Verification items for the finished model (mm, model axes). Face numbers are marked on the shaded views. A direction names the side the tool comes from. Coordinates: 2 decimals unless noted, no trailing zeros. Order: outer loops, then holes, each group sorted by start corner. A loop starts at its lowest first (then second) coordinate and runs counter-clockwise, first axis right, second up. Notation, with made-up numbers: M -38,20 L 18,20 A6 ccw 18,31 Z; hole C 88.5,45.25 d3. An arc over 180 degrees is marked long. Return JSON: item names as keys, results as strings. Group by question number.
Q1. Section check C-C, the plane z = 15.5. Enter the section's corners in (x, y), then the cut area to 3 significant figures.
Q2. Thickness scan on probe 1 along X at (y, z) = (-7, 20.5); probe 2 along X at (y, z) = (-21.5, 28); probe 3 along Z at (x, y) = (-29, -13). Record the ranges inside material, lowest first.
Q3. Section check B-B, the plane x = -28. Enter the section's corners in (y, z), then the cut area to 3 significant figures.
Q4. Section check D-D, the plane x = -24. Enter the section's corners in (y, z), then the cut area to 3 significant figures.
Q5. Mould release check, pull along X, two halves, no side actions. Record for the marked faces 1, 2 and 3: pulls with the +X half, pulls with the -X half, needs draft (parallel to the pull), parting line crosses it, or undercut.
Q6. Section check A-A, the plane y = -18. Enter the section's corners in (x, z), then the cut area to 3 significant figures.
Q7. Go/stop test with flat-tipped pins: pin 1 Ø4 at (x, z) = (-14, 7.5) entering from +Y; pin 2 Ø19.5 at (y, z) = (-38.5, 24) entering from +X; pin 3 Ø1 at (y, z) = (-32, 13.5) entering from +X; pin 4 Ø2 at (x, z) = (-24.5, 5.5) entering from -Y. Record where each tip stops, or that it passes through.
Q8. Access from +Z, -Z, +X, -X, +Y, -Y to the whole of each face (thin tool, end or side, straight path). Record for the marked faces 4, 5 and 6.
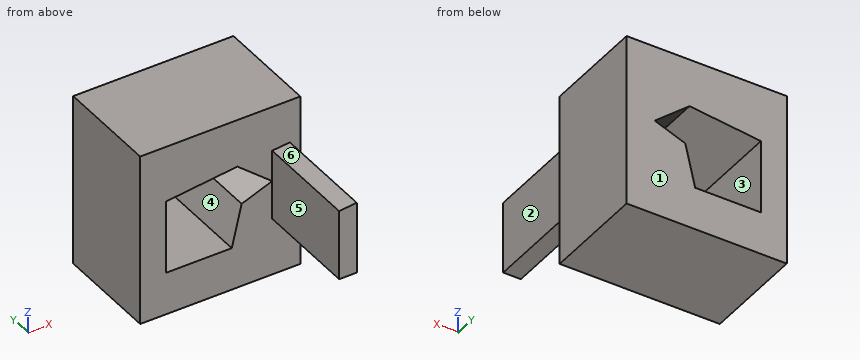
from build123d import *

# Parameters (mm, degrees)
F0_W     = 39.1931459308
F0_H     = 42.3528775573
F1_DEPTH = 25.4
F3_DEPTH = 25.4
F5_DEPTH = 25.4


# Not quite as in the source:
# - ends of sketch curves that miss each other by under 0.0002 mm in the source are joined
# - a feature of the source that left no trace in its solid (it failed there, or was rolled back) is left out


with BuildPart() as f1:
    # F0 (on Front) → F1 (new body)
    with BuildSketch(Plane.XZ):
        with Locations((-19.5965729654, 21.1764387786)):
            Rectangle(F0_W, F0_H)
    extrude(amount=F1_DEPTH)

    # F2 (on face) → F3 (cut)
    with BuildSketch(Plane.XZ.offset(25.4)):
        Polygon((-6.8881497718, 23.612594232), (-15.3977563605, 30.5856615305), (-32.8769646585, 28.529709205), (-32.8769646585, 10.48855111), (-16.7776942253, 10.48855111), (-14.3628085498, 20.764878951), align=None)
        Polygon((-21.8374673277, 17.9171636701), (-14.3628085498, 20.764878951), (-20.9175087512, 15.6267150305), align=None, mode=Mode.SUBTRACT)
        Polygon((-20.9175087512, 15.6267150305), (-14.3628085498, 20.764878951), (-21.8374673277, 17.9171636701), align=None)
    extrude(amount=-F3_DEPTH, mode=Mode.SUBTRACT)

    # F4 (on face) → F5 (join)
    with BuildSketch(Plane.XZ.offset(25.4)):
        Polygon((-6.8881497718, 31.2989987433), (-6.8881497718, 23.612594232), (-6.8881497718, 14.083658345), (-2.5741870049, 14.083658345), (-2.5741870049, 31.7389145494), align=None)
    extrude(amount=F5_DEPTH)


solid = f1.part
Numbers:
{
 "1": {"outline": "M -39.19,-25.4 L -32.88,-25.4 L -32.88,0 L -39.19,0 Z; M -15.6,-25.4 L -6.89,-25.4 L -6.89,-50.8 L -2.57,-50.8 L -2.57,-25.4 L 0,-25.4 L 0,0 L -15.6,0 Z", "area": "666 mm2"},
 "2": {"probe 1": "x = -39.19 to -32.88, -14.43 to 0", "probe 2": "x = -39.19 to -32.88, -12.24 to 0", "probe 3": "z = 0 to 10.49, 28.99 to 42.35"},
 "3": {"outline": "M -25.4,0 L 0,0 L 0,10.49 L -25.4,10.49 Z; M -25.4,29.1 L 0,29.1 L 0,42.35 L -25.4,42.35 Z", "area": "603 mm2"},
 "4": {"outline": "M -25.4,0 L 0,0 L 0,10.49 L -25.4,10.49 Z; M -25.4,29.57 L 0,29.57 L 0,42.35 L -25.4,42.35 Z", "area": "591 mm2"},
 "5": {"face 1": "needs draft", "face 2": "pulls with the +X half", "face 3": "undercut"},
 "6": {"outline": "M -39.19,0 L 0,0 L 0,42.35 L -39.19,42.35 Z; hole M -32.88,10.49 L -16.78,10.49 L -14.36,20.76 L -6.89,23.61 L -15.4,30.59 L -32.88,28.53 Z", "area": "1,290 mm2"},
 "7": {"pin 1": "stops at y = 0", "pin 2": "stops at x = -2.57", "pin 3": "passes through", "pin 4": "stops at y = -25.4"},
 "8": {"face 4": "+Y, -Y", "face 5": "+Z, -Z, -X, -Y", "face 6": "+Z, -X, -Y"}
}
